```python
from build123d import *

# Parameters (mm, degrees)
F0_W     = 3
F0_H     = 20
F1_DEPTH = 6.5
F2_DEPTH = 3
F3_DEPTH = 3


# Not quite as in the source:
# - a feature names something its author has since deleted; it is built from what else it names


with BuildPart() as f1:
    # F0 (on Top) → F1 (new body)
    with BuildSketch(Plane.XY):
        with Locations((-1.5, 10)):
            Rectangle(F0_W, F0_H)
        Polygon((-27, 0), (-3, 0), (-3, 20), (-15, 20), (-27, 20), align=None)
        with BuildLine():
            Line((-17, 11.5), (-15, 11.5))
            Line((-15, 11.5), (-13, 11.5))
            Line((-13, 11.5), (-11.5, 11.5))
            ThreePointArc((-11.5, 11.5), (-10.0857864376, 10.9142135624), (-9.5, 9.5))
            ThreePointArc((-9.5, 9.5), (-10.0857864376, 8.0857864376), (-11.5, 7.5))
            Line((-11.5, 7.5), (-13, 7.5))
            Line((-13, 7.5), (-17, 7.5))
            Line((-17, 7.5), (-18.5, 7.5))
            ThreePointArc((-18.5, 7.5), (-20.5, 9.5), (-18.5, 11.5))
            Line((-18.5, 11.5), (-17, 11.5))
        make_face(mode=Mode.SUBTRACT)
        with Locations((-28.5, 10)):
            Rectangle(F0_W, F0_H)
        with BuildLine():
            Line((-17, 10.8228756555), (-17, 11.5))
            Line((-17, 11.5), (-18.5, 11.5))
            ThreePointArc((-18.5, 11.5), (-17.6771243445, 11.3228756555), (-17, 10.8228756555))
        make_face()
        with BuildLine():
            Line((-11.5, 11.5), (-13, 11.5))
            Line((-13, 11.5), (-13, 10.8228756555))
            ThreePointArc((-13, 10.8228756555), (-12.3228756555, 11.3228756555), (-11.5, 11.5))
        make_face()
        with BuildLine():
            ThreePointArc((-17, 10.8228756555), (-17.6771243445, 11.3228756555), (-18.5, 11.5))
            ThreePointArc((-18.5, 11.5), (-20.5, 9.5), (-18.5, 7.5))
            Line((-18.5, 7.5), (-17, 7.5))
            Line((-17, 7.5), (-17, 9.5))
            Line((-17, 9.5), (-17, 10.8228756555))
        make_face()
        with BuildLine():
            ThreePointArc((-9.5, 9.5), (-10.0857864376, 10.9142135624), (-11.5, 11.5))
            ThreePointArc((-11.5, 11.5), (-12.3228756555, 11.3228756555), (-13, 10.8228756555))
            Line((-13, 10.8228756555), (-13, 8.1771243445))
            ThreePointArc((-13, 8.1771243445), (-12.3228756555, 7.6771243445), (-11.5, 7.5))
            ThreePointArc((-11.5, 7.5), (-10.0857864376, 8.0857864376), (-9.5, 9.5))
        make_face()
        with BuildLine():
            ThreePointArc((-11.5, 7.5), (-12.3228756555, 7.6771243445), (-13, 8.1771243445))
            Line((-13, 8.1771243445), (-13, 7.5))
            Line((-13, 7.5), (-11.5, 7.5))
        make_face()
    extrude(amount=F1_DEPTH)

    # F0 (on Top) → F2 (join)
    with BuildSketch(Plane.XY):
        with Locations((-1.5, 10)):
            Rectangle(F0_W, F0_H)
        with Locations((-28.5, 10)):
            Rectangle(F0_W, F0_H)
        with BuildLine():
            Line((-17, 10.8228756555), (-17, 11.5))
            Line((-17, 11.5), (-18.5, 11.5))
            ThreePointArc((-18.5, 11.5), (-17.6771243445, 11.3228756555), (-17, 10.8228756555))
        make_face()
        with BuildLine():
            Line((-11.5, 11.5), (-13, 11.5))
            Line((-13, 11.5), (-13, 10.8228756555))
            ThreePointArc((-13, 10.8228756555), (-12.3228756555, 11.3228756555), (-11.5, 11.5))
        make_face()
        with BuildLine():
            ThreePointArc((-17, 10.8228756555), (-17.6771243445, 11.3228756555), (-18.5, 11.5))
            ThreePointArc((-18.5, 11.5), (-20.5, 9.5), (-18.5, 7.5))
            Line((-18.5, 7.5), (-17, 7.5))
            Line((-17, 7.5), (-17, 9.5))
            Line((-17, 9.5), (-17, 10.8228756555))
        make_face()
        with BuildLine():
            ThreePointArc((-9.5, 9.5), (-10.0857864376, 10.9142135624), (-11.5, 11.5))
            ThreePointArc((-11.5, 11.5), (-12.3228756555, 11.3228756555), (-13, 10.8228756555))
            Line((-13, 10.8228756555), (-13, 8.1771243445))
            ThreePointArc((-13, 8.1771243445), (-12.3228756555, 7.6771243445), (-11.5, 7.5))
            ThreePointArc((-11.5, 7.5), (-10.0857864376, 8.0857864376), (-9.5, 9.5))
        make_face()
        with BuildLine():
            ThreePointArc((-11.5, 7.5), (-12.3228756555, 7.6771243445), (-13, 8.1771243445))
            Line((-13, 8.1771243445), (-13, 7.5))
            Line((-13, 7.5), (-11.5, 7.5))
        make_face()
    extrude(amount=-F2_DEPTH)

    # F0 (on Top) → F3 (join)
    with BuildSketch(Plane.XY):
        with Locations((-28.5, 10)):
            Rectangle(F0_W, F0_H)
        with Locations((-1.5, 10)):
            Rectangle(F0_W, F0_H)
    extrude(amount=-F3_DEPTH)


solid = f1.part
```
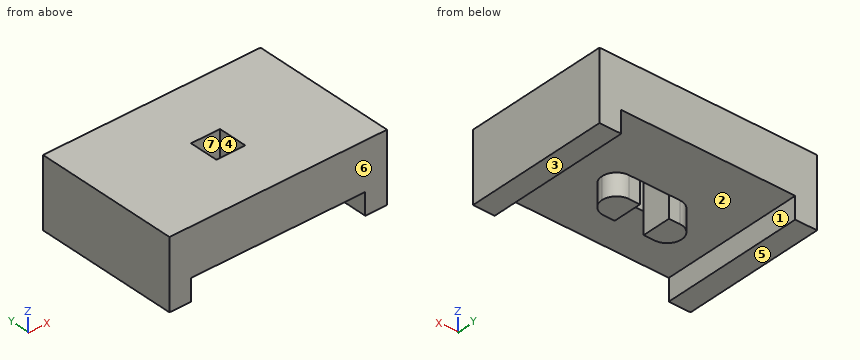
Part model, mm, in its own coordinate system. Face numbers are marked on the shaded views. A direction names the side the tool comes from. Give positions to 0.01 mm unless a question says otherwise; leave off trailing zeros. Order: outer loops, then holes, each group sorted by start corner. A loop starts at its lowest first (then second) coordinate and runs counter-clockwise, first axis right, second up. Notation, with made-up numbers: (11.25, 56.5) - (35.25, 56.5) arc R24 cw to (35.25, 85.5) - close; hole circle Ø5 at (-37.5, 68.25). An arc over 180 degrees is marked (long way). Use one line per item in the form item = value.
Item 1: Probe probe 1 along X at (y, z) = (10.75, -1.25); probe 2 along X at (y, z) = (11, 5.75); probe 3 along Z at (x, y) = (-12, 19). List the from-to ranges inside material, lowest first. Write a range as from..to.
Solution:
probe_1 = -30..-27, -20.06..-17, -13..-9.94, -3..0
probe_2 = -30..-17, -13..0
probe_3 = 0..6.5
Item 2: Slice it at A-A on y = 10.75. Give the cut face in (x, z).
Solution:
outline = (-30, -3) - (-27, -3) - (-27, 0) - (-20.06, 0) - (-20.06, -3) - (-17, -3) - (-17, 6.5) - (-30, 6.5) - close; (-13, -3) - (-9.94, -3) - (-9.94, 0) - (-3, 0) - (-3, -3) - (0, -3) - (0, 6.5) - (-13, 6.5) - close
Item 3: Slice it at D-D on y = 5.25. Give the cut face in (x, z).
Solution:
outline = (-30, -3) - (-27, -3) - (-27, 0) - (-3, 0) - (-3, -3) - (0, -3) - (0, 6.5) - (-30, 6.5) - close
Item 4: Two-plate mould, pull along Y, no slides. Class the marked faces 5, 6 and 7: released by +Y, released by -Y, zero draft, split by the parting line, or undercut.
Solution:
face_5 = zero draft
face_6 = released by -Y
face_7 = undercut
Item 5: Pin check, flat tips, straight feed: pin 1 Ø0.8 at (x, z) = (-12, -1) entering from -Y; pin 2 Ø0.8 at (x, z) = (-12.5, -2) entering from +Y; pin 3 Ø2 at (x, z) = (-25.5, -2) entering from -Y. Stop position of each tip, or through.
Solution:
pin_1 = 7.5
pin_2 = 11.5
pin_3 = through
Item 6: Slice it at C-C on z = 4.25. Give the cut face in (x, y), and give its area (3 significant figures).
Solution:
outline = (-30, 0) - (0, 0) - (0, 20) - (-30, 20) - close; hole (-17, 7.5) - (-13, 7.5) - (-13, 11.5) - (-17, 11.5) - close
area = 584 mm2
Item 7: Which spindle directions (+Z, -Z, +X, -X, +Y, -Y) get a long thin tool onto all of the face, cutting with end or side? Do the marked faces 1, 2, 3 and 4. Say none if no direction does.
Solution:
face_1 = -Z, +Y, -Y
face_2 = -Z
face_3 = -Z, +X, -X, +Y, -Y
face_4 = +Z, -Z
Item 8: Slice it at B-B on x = -14.5. Give the cut face in (y, z), and give its area (3 significant figures).
Solution:
outline = (0, 0) - (7.5, 0) - (7.5, 6.5) - (0, 6.5) - close; (11.5, 0) - (20, 0) - (20, 6.5) - (11.5, 6.5) - close
area = 104 mm2
